Design review of the part shown in the three views and the two pictorial views. Dimensions are in mm from the part's minimum x, y and z. A direction names the side the tool comes from. Coordinates: 2 decimals unless noted, no trailing zeros. Write each loop counter-clockwise with the first axis right and the second up, starting at its lowest first coordinate (ties: lowest second). Pieces come first, ordered by that corner, then holes. Notation, with made-up numbers: (45, 47.25) - (92, 47.25) arc R11 cw to (92, 58.25) - close; hole circle Ø8 at (74.25, 85.25). An arc over 180 degrees is marked (long way). Write each question's results on one line, items separated by ' | '.
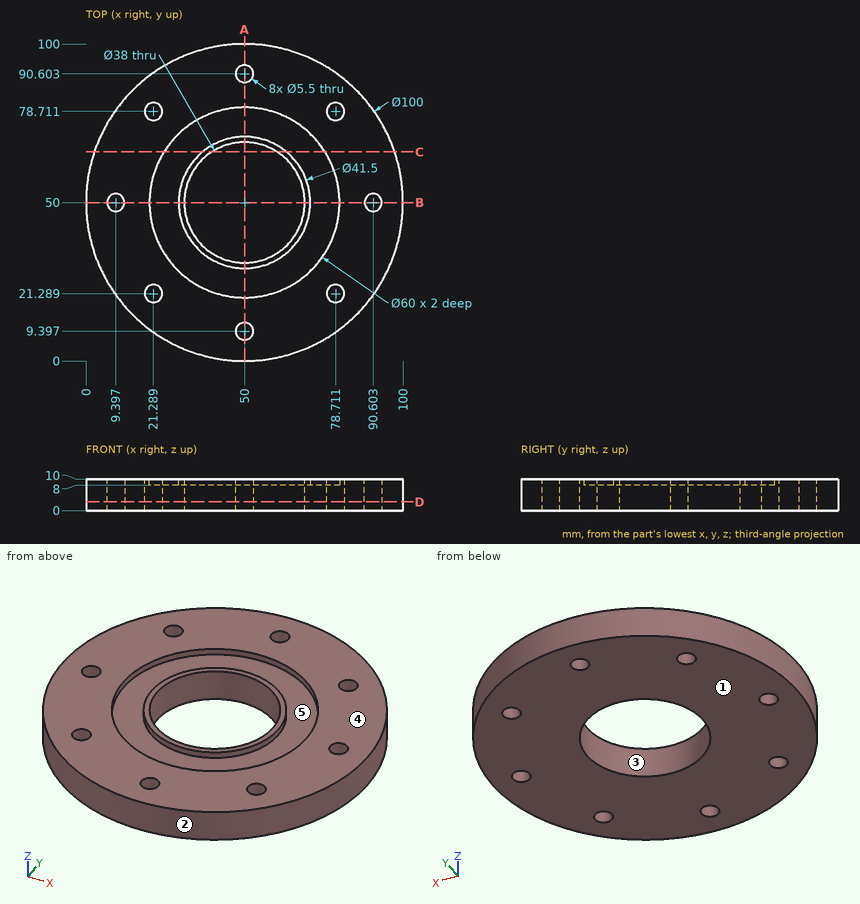
Q1. Take a section at C-C on y = 66. State the section outline as (x, z) points, plus the area to 3 significant figures.
Results found:
outline: (2.63, 0) - (39.75, 0) - (39.75, 10) - (36.79, 10) - (36.79, 8) - (24.62, 8) - (24.62, 10) - (2.63, 10) - close; (60.25, 0) - (97.37, 0) - (97.37, 10) - (75.38, 10) - (75.38, 8) - (63.21, 8) - (63.21, 10) - (60.25, 10) - close | area: 694 mm2
Q2. For the marked faces 4 and 5, list the 3-axis set-ups (+Z, -Z, +X, -X, +Y, -Y) from which the entire face can be reached by the end or side of a thin tool; tool diameter is ignored.
Results found:
face 4: +Z, +X, -X, +Y, -Y | face 5: +Z
Q3. Take a section at D-D on z = 2.75. State how many separate pieces and enclosed holes the cut face has, plus the area to 3 significant figures.
Results found:
separate pieces: 1 | enclosed holes: 9 | area: 6,530 mm2
Q4. Wall thickness on line 1 along Y through (x, z) = (50, 0.75); line 2 along Y through (x, z) = (52, 8.5) (1 decimal); line 3 along Z through (x, y) = (28.5, 68): over which ranges is each line inside the solid? List them lowest first. Write a range as from..to.
Results found:
line 1: 0..6.65, 12.15..31, 69..87.85, 93.35..100 | line 2: 0..7.5, 11.3..20.1, 29.3..31.1, 68.9..70.7, 79.9..88.7, 92.5..100 | line 3: 0..8
Q5. Take a section at A-A on x = 50. State the section outline as (y, z) points.
Results found:
outline: (0, 0) - (6.65, 0) - (6.65, 10) - (0, 10) - close; (12.15, 0) - (31, 0) - (31, 10) - (29.25, 10) - (29.25, 8) - (20, 8) - (20, 10) - (12.15, 10) - close; (69, 0) - (87.85, 0) - (87.85, 10) - (80, 10) - (80, 8) - (70.75, 8) - (70.75, 10) - (69, 10) - close; (93.35, 0) - (100, 0) - (100, 10) - (93.35, 10) - close
Q6. For pin 1 (6 mm diameter, centred on x = 36.5, z = 3, fed in from +Y) (1 decimal); pin 2 (5 mm diameter, centred on x = 82, z = 4.5, fed in from -Y); pin 3 (7 mm diameter, centred on x = 50, y = 9.4, fed in from -Z); pin 4 (5 mm diameter, centred on y = 62, z = 7, fed in from +X), all flat-tipped, find the tip position at first contact; note any pin that passes through.
Results found:
pin 1: y = 98.9 | pin 2: y = 9.63 | pin 3: z = 0 | pin 4: x = 99.09
Q7. Mouldability with a two-part tool opening along Y and no side actions: class the marked faces 1, 2 and 3 as pulls with the +Y half, pulls with the -Y half, needs draft (parallel to the pull), parting line crosses it, or undercut.
Results found:
face 1: needs draft | face 2: parting line crosses it | face 3: undercut
